Source: CAD feature listing. Evaluate the final solid. Frame: model axes, mm. A direction names the side the tool comes from. Coordinates: 2 decimals unless noted, no trailing zeros. Write each loop counter-clockwise with the first axis right and the second up, starting at its lowest first coordinate (ties: lowest second). Pieces come first, ordered by that corner, then holes. Notation, with made-up numbers: (75, -40) - (110, -40) arc R11 ccw to (110, -34) - close; hole circle Ø3 at (31, 37.25). An arc over 180 degrees is marked (long way). One line per item, written item: value.
from build123d import *

# Parameters (mm, degrees)
F0_R        = 38
F0_R_2      = 4
F1_DEPTH    = 10
F3_R        = 5
F1_FACE_R   = 38
F1_FACE_R_2 = 4
F4_DEPTH    = 12
F5_R        = 18
F6_DEPTH    = 48
F7_W        = 18.915552
F7_H        = 85.689727
F8_DEPTH    = 40
F9_R        = 13
F10_DEPTH   = 25
F11_R       = 10
F12_DEPTH   = 45.001
F13_R       = 2
F14_SIZE    = 2


with BuildPart() as f1:
    # F0 (on Front) → F1 (new body)
    with BuildSketch(Plane.XZ):
        Circle(F0_R)
        with Locations((-25.114737, -14.5)):
            Circle(F0_R_2, mode=Mode.SUBTRACT)
        with Locations((0, -29)):
            Circle(F0_R_2, mode=Mode.SUBTRACT)
        with Locations((25.114737, -14.5)):
            Circle(F0_R_2, mode=Mode.SUBTRACT)
        with Locations((-25.114737, 14.5)):
            Circle(F0_R_2, mode=Mode.SUBTRACT)
        with Locations((25.114737, 14.5)):
            Circle(F0_R_2, mode=Mode.SUBTRACT)
        with Locations((0, 29)):
            Circle(F0_R_2, mode=Mode.SUBTRACT)
    extrude(amount=F1_DEPTH)

    # F3 (on offset) + F1_face (on face) → F4 (join)
    with BuildSketch(Plane.XZ.offset(70)):
        with BuildLine():
            Line((11.27594, -42.105263), (23.491541, -8.552632))
            ThreePointArc((23.491541, -8.552632), (25, 0), (23.491541, 8.552632))
            Line((23.491541, 8.552632), (11.27594, 42.105263))
            ThreePointArc((11.27594, 42.105263), (0, 50), (-11.27594, 42.105263))
            Line((-11.27594, 42.105263), (-23.491541, 8.552632))
            ThreePointArc((-23.491541, 8.552632), (-25, 0), (-23.491541, -8.552632))
            Line((-23.491541, -8.552632), (-11.27594, -42.105263))
            ThreePointArc((-11.27594, -42.105263), (0, -50), (11.27594, -42.105263))
        make_face()
        with Locations((0, -38)):
            Circle(F3_R, mode=Mode.SUBTRACT)
        with Locations((0, 38)):
            Circle(F3_R, mode=Mode.SUBTRACT)
    with BuildSketch(Plane.XZ.offset(10)):
        Circle(F1_FACE_R)
        with Locations((-25.114737, -14.5)):
            Circle(F1_FACE_R_2, mode=Mode.SUBTRACT)
        with Locations((0, -29)):
            Circle(F1_FACE_R_2, mode=Mode.SUBTRACT)
        with Locations((25.114737, -14.5)):
            Circle(F1_FACE_R_2, mode=Mode.SUBTRACT)
        with Locations((-25.114737, 14.5)):
            Circle(F1_FACE_R_2, mode=Mode.SUBTRACT)
        with Locations((25.114737, 14.5)):
            Circle(F1_FACE_R_2, mode=Mode.SUBTRACT)
        with Locations((0, 29)):
            Circle(F1_FACE_R_2, mode=Mode.SUBTRACT)
    extrude(amount=-F4_DEPTH)

    # F5 (on face) → F6 (join, through all)
    with BuildSketch(Plane.XZ.offset(10)):
        Circle(F5_R)
    extrude(amount=F6_DEPTH)

    # F7 (on Right) → F8 (cut, symmetric)
    with BuildSketch(Plane.YZ):
        with Locations((9.457776, 1.025541)):
            Rectangle(F7_W, F7_H)
    extrude(amount=F8_DEPTH, both=True, mode=Mode.SUBTRACT)

    # F9 (on face) → F10 (cut)
    with BuildSketch(Plane(origin=(0, 0, 0), x_dir=(-1, 0, 0), z_dir=(0, 1, 0))):
        Circle(F9_R)
    extrude(amount=-F10_DEPTH, mode=Mode.SUBTRACT)

    # F11 (on face) → F12 (cut, through all)
    with BuildSketch(Plane(origin=(0, -25, 0), x_dir=(-1, 0, 0), z_dir=(0, 1, 0))):
        Circle(F11_R)
    extrude(amount=-F12_DEPTH, mode=Mode.SUBTRACT)

    # F13
    f13_edges = [f1.edges().sort_by_distance(p)[0] for p in [
        (-18, -58, 0),
        (17.38374, -58, 25.328947),
        (-18, -10, 0),
        (-38, -10, 0),
    ]]
    fillet(f13_edges, radius=F13_R)

    # F14
    f14_edges = [f1.edges().sort_by_distance(p)[0] for p in [
        (10, -70, 0),
    ]]
    chamfer(f14_edges, length=F14_SIZE)


solid = f1.part
1) Draft query along Z for faces 4 (the cylindrical face through (16.73, -58.57, 25.36)), 5 (the cylindrical face through (-16.73, -58.57, -25.36)), 6 (the flat face through (-7, -25, -8)). Return one class per face: released by +Z, released by -Z, zero draft, split by the parting line, or undercut.
Values found:
face 4: released by +Z
face 5: released by -Z
face 6: undercut
2) Section query C-C on y = -35.5. Output: boundary loops of the cut face in (x, z).
Values found:
outline: circle Ø36 at (0, 0); hole circle Ø20 at (0, 0)
3) Section query B-B on x = 0. State how many separate pieces and enclosed holes the cut face has, then the cut area to 3 significant figures.
Values found:
separate pieces: 6
enclosed holes: 0
area: 1,730 mm2
4) Contact query for flat-ended pins moving along their axis: P1, Ø5, axis at y = -45.5, z = 1.5, coming from the -X side; P2, Ø8, axis at x = 1, z = 6.5, coming from the +Y side; P3, Ø12, axis at y = -56, z = 25, coming from the -X side. Output: stop coordinate, or through.
Values found:
P1: x = -18
P2: y = -25
P3: x = -19.21
5) Material intervals for line 1 (Z direction, x = 0, y = -6.75); line 2 (Z direction, x = 0, y = -63.5); line 3 (Y direction, x = 19.5, z = 8), sorted ascending.
Values found:
line 1: -38 to -33, -25 to -13, 13 to 25, 33 to 38
line 2: -50 to -43, -33 to -10, 10 to 33, 43 to 50
line 3: -70 to -58, -10 to 0
6) Reachability of faces 1 (the cylindrical face through (28.93, -4.93, 15.7)), 2 (the cylindrical face through (3, -64, -34)), 3 (the cylindrical face through (-25, -65, 0)) from +Z, -Z, +X, -X, +Y, -Y: full face, straight path, thin tool, end or side. Return the list, or none.
Values found:
face 1: +Y
face 2: -Y
face 3: -X, -Y
